```python
from build123d import *

# Parameters (mm, degrees)
F0_R     = 4.3688
F1_DEPTH = 28.4226
F0_R_2   = 7.62
F2_DEPTH = 2.54
F3_R     = 3.175
F4_DEPTH = 30.9636


# Not quite as in the source:
# - a feature names something its author has since deleted; it is built from what else it names


with BuildPart() as f1:
    # F0 (on Top) → F1 (new body)
    with BuildSketch(Plane.XY):
        Circle(F0_R)
    extrude(amount=F1_DEPTH)

    # F0 (on Top) → F2 (join)
    with BuildSketch(Plane.XY):
        Circle(F0_R_2)
        Circle(F0_R, mode=Mode.SUBTRACT)
        Circle(F0_R)
    extrude(amount=-F2_DEPTH)

    # F3 (on face) → F4 (cut, through all)
    with BuildSketch(Plane.XY.offset(28.4226)):
        Circle(F3_R)
    extrude(amount=-F4_DEPTH, mode=Mode.SUBTRACT)


solid = f1.part
```
Build history of the part. All positions in model axes, mm. Round coordinates to 2 decimals unless told otherwise and drop trailing zeros. Loops run counter-clockwise (first coordinate to the right, second up) from the corner with the lowest first, then second, coordinate; pieces in that order, holes last.
Item 1: Saw through at C-C (z = 3). List the corners of the cut face in (x, y) (3 decimals), then the cut area to 3 significant figures.
Item 2: Saw through at A-A (x = 0). List the corners of the cut face in (y, z) (3 decimals), then the cut area to 3 significant figures.
Item 3: Pin check, flat tips, straight feed: P1, Ø5, axis at y = -2, z = 10.5, coming from the -X side; P2, Ø1.5, axis at x = 2, z = 20, coming from the -Y side; P3, Ø5, axis at y = -4, z = 24.5, coming from the +X side. Stop position of each tip, or through.
Item 4: Saw through at D-D (y = -5.5). List the corners of the cut face in (x, z), then the cut area to 3 significant figures.
Item 5: Two-plate mould, pull along Y, no slides. Class faces 1 (the face through (4.167, 1.312, 14.012)), 2 (the face through (3.3, -3.3, 0)), 3 (the face through (-0.69, -3.1, 13.16)): released by +Y, released by -Y, zero draft, split by the parting line, or undercut.
Item 6: Drill centre lines: line 1 along Y through (x, z) = (0, 20.5) (3 decimals); line 2 along Z through (x, y) = (1.75, -6.5); line 3 along Y through (x, z) = (-1, 25.5). Where is each one in solid material? Low to high.
Worked answers:
1. outline: circle Ø8.738 at (0, 0); hole circle Ø6.35 at (0, 0)
1. area: 28.3 mm2
2. outline: (-7.62, -2.54) - (-3.175, -2.54) - (-3.175, 28.423) - (-4.369, 28.423) - (-4.369, 0) - (-7.62, 0) - close; (3.175, -2.54) - (7.62, -2.54) - (7.62, 0) - (4.369, 0) - (4.369, 28.423) - (3.175, 28.423) - close
2. area: 90.4 mm2
3. P1: stops at x = -4.37
3. P2: stops at y = -4.19
3. P3: stops at x = 4.1
4. outline: (-5.27, -2.54) - (5.27, -2.54) - (5.27, 0) - (-5.27, 0) - close
4. area: 26.8 mm2
5. face 1: split by the parting line
5. face 2: zero draft
5. face 3: undercut
6. line 1: y = -4.369 to -3.175, 3.175 to 4.369
6. line 2: z = -2.54 to 0
6. line 3: y = -4.25 to -3.01, 3.01 to 4.25
